Design review of the part built by this model. Coordinates are the model's own, in mm. A direction names the side the tool comes from. Coordinates: 2 decimals unless noted, no trailing zeros. Write each loop counter-clockwise with the first axis right and the second up, starting at its lowest first coordinate (ties: lowest second). Pieces come first, ordered by that corner, then holes.
Q1. Add section D-D, the plane y = 23. Give the boundary of the cut face in (x, z), plus the area to 3 significant figures.
Q2. Add section A-A, the plane z = 0.75. Give the boundary of the cut face in (x, y).
Q3. Add section B-B, the plane y = 10.5. Give the boundary of the cut face in (x, z).
Q4. Clearance check with flat-ended pins moving along their axes: pin 1 Ø0.8 at (x, y) = (-1.5, -1) entering from +Z; pin 2 Ø8 at (x, z) = (4, -4) entering from +Y; pin 3 Ø1.6 at (y, z) = (-0.5, 1) entering from -X; pin 4 Ø1.6 at (x, y) = (0.5, -0.5) entering from -Z. State where each tip first meets the part, or that it passes through.
Q5. To check wall thickness, follow probe 1 along Z at (x, y) = (-3.75, 1.5); probe 2 along Y at (x, z) = (-5.5, -8); probe 3 along Z at (x, y) = (-1.5, 20.5). State the ranges of each line that lie inside material, in increasing order.
Q6. Machinability: for faces 1 (the face through (2, 5.5, -10.7)), 2 (the face through (0, -1, 6)), 3 (the face through (0, -1, -6)), 4 (the face through (6, -1, 0)), 5 (the face through (2, 14.5, 1)), which of the approach directions +Z, -Z, +X, -X, +Y, -Y give a long, thin tool a straight path to every point of the face, cutting with its end or side? Answer none if there is none.
Q7. Add section C-C, the plane z = -7.75. Give the boundary of the cut face in (x, y).
from build123d import *

# Parameters (mm, degrees)
SKETCH1_W           = 16.2
SKETCH1_H           = 17.5
BOSS_EXTRUDE1_DEPTH = 6
SKETCH2_W           = 12
SKETCH2_H           = 12
BOSS_EXTRUDE2_DEPTH = 1.5
SKETCH3_R           = 4.5
BOSS_EXTRUDE3_DEPTH = 7
SKETCH4_R           = 3
BOSS_EXTRUDE4_DEPTH = 13.5
CUT_EXTRUDE1_DEPTH  = 12
SKETCH6_W           = 4
SKETCH6_H           = 1
BOSS_EXTRUDE5_DEPTH = 3
FILLET1_R           = 1
CHAMFER1_SIZE       = 1.5
CHAMFER1_SIZE2      = 1
CHAMFER2_SIZE       = 1
CHAMFER2_SIZE2      = 1.5
BOSS_EXTRUDE6_DEPTH = 2.5
FILLET2_R           = 1


with BuildPart() as part:
    # Sketch1 → Boss-Extrude1 (new body)
    with BuildSketch(Plane(origin=(0, 0, 0), x_dir=(1, 0, 0), z_dir=(0, 1, 0))):
        Rectangle(SKETCH1_W, SKETCH1_H)
    extrude(amount=BOSS_EXTRUDE1_DEPTH)

    # Sketch2 → Boss-Extrude2 (add)
    with BuildSketch(Plane.XZ):
        Rectangle(SKETCH2_W, SKETCH2_H)
    extrude(amount=BOSS_EXTRUDE2_DEPTH)

    # Sketch3 → Boss-Extrude3 (add)
    with BuildSketch(Plane(origin=(0, 6, 0), x_dir=(1, 0, 0), z_dir=(0, 1, 0))):
        with Locations((0, -0.75)):
            Circle(SKETCH3_R)
    extrude(amount=BOSS_EXTRUDE3_DEPTH)

    # Sketch4 → Boss-Extrude4 (add)
    with BuildSketch(Plane(origin=(0, 13, 0), x_dir=(1, 0, 0), z_dir=(0, 1, 0))):
        with Locations((0, -0.75)):
            Circle(SKETCH4_R)
    extrude(amount=BOSS_EXTRUDE4_DEPTH)

    # Sketch5 → Cut-Extrude1 (cut)
    with BuildSketch(Plane(origin=(0, 26.5, 0), x_dir=(1, 0, 0), z_dir=(0, 1, 0))):
        with BuildLine():
            ThreePointArc((3, -0.75), (2.598076211, 0.75), (1.5, 1.848076211))
            Line((1.5, 1.848076211), (1.5, -3.348076211))
            ThreePointArc((1.5, -3.348076211), (2.598076211, -2.25), (3, -0.75))
        make_face()
    extrude(amount=-CUT_EXTRUDE1_DEPTH, mode=Mode.SUBTRACT)

    # Sketch6 → Boss-Extrude5 (add)
    with BuildSketch(Plane(origin=(0, 0, -8.75), x_dir=(-1, 0, 0), z_dir=(0, 0, -1))):
        with Locations((0, 5.5)):
            Rectangle(SKETCH6_W, SKETCH6_H)
    extrude(amount=BOSS_EXTRUDE5_DEPTH)

    # Fillet1
    fillet1_edges = [part.edges().sort_by_distance(p)[0] for p in [
        (-2, 5.5, -8.75),
        (2, 5.5, -8.75),
    ]]
    fillet(fillet1_edges, radius=FILLET1_R)

    # Chamfer1
    chamfer1_edges = [part.edges().sort_by_distance(p)[0] for p in [
        (-3, 26.5, 0.75),
    ]]
    chamfer1_side = [part.faces().sort_by_distance(p)[0] for p in [
        (-3, 19.75, 0.75),
    ]]
    chamfer(chamfer1_edges, length=CHAMFER1_SIZE, length2=CHAMFER1_SIZE2, reference=chamfer1_side[0])

    # Chamfer2
    chamfer2_edges = [part.edges().sort_by_distance(p)[0] for p in [
        (1.5, 26.5, 0.75),
    ]]
    chamfer2_side = [part.faces().sort_by_distance(p)[0] for p in [
        (-0.132366073, 26.5, 0.75),
    ]]
    chamfer(chamfer2_edges, length=CHAMFER2_SIZE, length2=CHAMFER2_SIZE2, reference=chamfer2_side[0])

    # Sketch7 → Boss-Extrude6 (add)
    with BuildSketch(Plane(origin=(0, 6, 0), x_dir=(1, 0, 0), z_dir=(0, 1, 0))):
        with BuildLine():
            Line((-1.5, 8.25), (1.5, 8.25))
            ThreePointArc((1.5, 8.25), (0, 9.75), (-1.5, 8.25))
        make_face()
    extrude(amount=BOSS_EXTRUDE6_DEPTH)

    # Fillet2
    fillet2_edges = [part.edges().sort_by_distance(p)[0] for p in [
        (0, 8.5, -9.75),
    ]]
    fillet(fillet2_edges, radius=FILLET2_R)


solid = part.part
Here are the results:
1. outline: (1.5, -1.85) - (1.5, 3.35) arc R3 ccw (long way) to start
1. area: 22.7 mm2
2. outline: (-8.1, 0) - (-6, 0) - (-6, -1.5) - (6, -1.5) - (6, 0) - (8.1, 0) - (8.1, 6) - (4.5, 6) - (4.5, 13) - (3, 13) - (3, 14.5) - (1.5, 14.5) - (1.5, 25) - (0.5, 26.5) - (-2, 26.5) - (-3, 25) - (-3, 13) - (-4.5, 13) - (-4.5, 6) - (-8.1, 6) - close
3. outline: circle Ø9 at (0, 0.75)
4. pin 1: stops at z = 6
4. pin 2: stops at y = 25.9
4. pin 3: stops at x = -8.1
4. pin 4: stops at z = -8.75
5. probe 1: z = -8.75 to 8.75
5. probe 2: y = 0 to 6
5. probe 3: z = -1.85 to 3.35
6. face 1: -Z, +X, +Y, -Y
6. face 2: +Z, +X, -X, -Y
6. face 3: -Z, +X, -X, -Y
6. face 4: +Z, -Z, +X, -Y
6. face 5: +Z, -Z, +X, +Y
7. outline: (-8.1, 0) - (8.1, 0) - (8.1, 6) - (-8.1, 6) - close
